```python
from build123d import *

# Parameters (mm, degrees)
ESBO_O6_W                = 100
ESBO_O6_H                = 400
RESSALTO_EXTRUS_O2_DEPTH = 18
CORTE_EXTRUS_O2_DEPTH    = 413.703283244
ESBO_O8_R                = 1.5
CORTE_EXTRUS_O3_DEPTH    = 413.703283244


with BuildPart() as part:
    # Esboço6 → Ressalto-extrusão2 (new body)
    with BuildSketch(Plane.XY):
        with Locations((50, 200)):
            Rectangle(ESBO_O6_W, ESBO_O6_H)
    extrude(amount=RESSALTO_EXTRUS_O2_DEPTH)

    # Esboço7 → Corte-extrusão2 (cut, through all)
    with BuildSketch(Plane.XY.offset(18)):
        Polygon((50, 400), (100, 350), (100, 400), align=None)
        Polygon((100, 50), (50, 0), (100, 0), align=None)
    extrude(amount=-CORTE_EXTRUS_O2_DEPTH, mode=Mode.SUBTRACT)

    # Esboço8 → Corte-extrusão3 (cut, through all)
    with BuildSketch(Plane(origin=(0, 0, 0), x_dir=(-1, 0, 0), z_dir=(0, 0, -1))):
        with Locations((-75, 160)):
            Circle(ESBO_O8_R)
        with Locations((-43, 160)):
            Circle(ESBO_O8_R)
        with Locations((-9, 50)):
            Circle(ESBO_O8_R)
        with Locations((-9, 110)):
            Circle(ESBO_O8_R)
    extrude(amount=-CORTE_EXTRUS_O3_DEPTH, mode=Mode.SUBTRACT)


solid = part.part
```
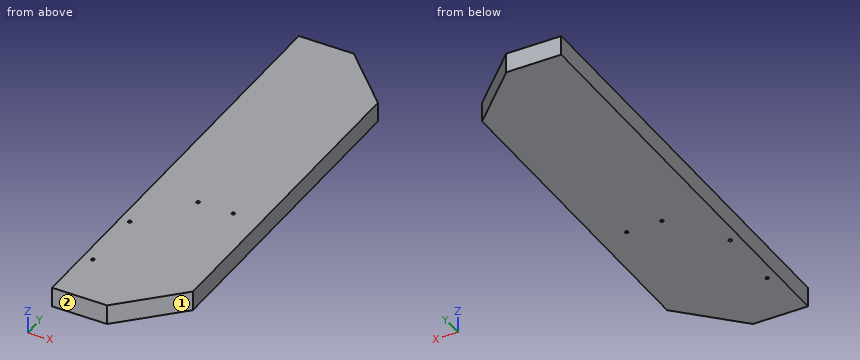
Can you work these out from the model? Positions are in its coordinate system, mm. Face numbers are marked on the shaded views. Coordinates: 2 decimals unless noted, no trailing zeros. Order: outer loops, then holes, each group sorted by start corner. A loop starts at its lowest first (then second) coordinate and runs counter-clockwise, first axis right, second up. Notation, with made-up numbers: (24.5, 76) - (31.5, 76) arc R15 ccw to (31.5, 97) - close; hole circle Ø9 at (-38, -28). An arc over 180 degrees is marked (long way). Answer in a Markdown table with one row per item.
1. Suppose I cut it at B-B (x = 86.5). Please give me the cut outline in (y, z).
Reply:
| item | result |
|---|---|
| outline | (36.5, 0) - (363.5, 0) - (363.5, 18) - (36.5, 18) - close |
2. If we mould it in two halves opening along X, with no side actions, what happens to the marked faces 1 and 2? For each: pulls with the +X half, pulls with the -X half, needs draft (parallel to the pull), parting line crosses it, or undercut.
Reply:
| item | result |
|---|---|
| face 1 | pulls with the +X half |
| face 2 | needs draft |
3. Suppose I cut it at A-A (z = 11.5). Please give me the cut outline in (x, y), and give its area (3 significant figures).
Reply:
| item | result |
|---|---|
| outline | (0, 0) - (50, 0) - (100, 50) - (100, 350) - (50, 400) - (0, 400) - close; hole circle Ø3 at (9, 50); hole circle Ø3 at (9, 110); hole circle Ø3 at (43, 160); hole circle Ø3 at (75, 160) |
| area | 37,500 mm^2 |
4. Suppose I cut it at C-C (x = 68). Please give me the cut outline in (y, z).
Reply:
| item | result |
|---|---|
| outline | (18, 0) - (382, 0) - (382, 18) - (18, 18) - close |
5. For pin 1 (4 mm diameter, centred on x = 63.5, z = 3.5, fed in from +Y); pin 2 (1.8 mm diameter, centred on x = 9, y = 50, fed in from -Z); pin 3 (3 mm diameter, centred on x = 81.5, z = 14, fed in from -Y), each with a flat end and sliding along its axis, tell me the tip position at first contact or that it passes through.
Reply:
| item | result |
|---|---|
| pin 1 | stops at y = 388.5 |
| pin 2 | passes through |
| pin 3 | stops at y = 30 |
6. If I drill on line 1 along X through (y, z) = (160, 7.5); line 2 along Y through (x, z) = (9, 17); line 3 along X through (y, z) = (110, 14), over which ranges is the centre line in solid material (lowest first)?
Reply:
| item | result |
|---|---|
| line 1 | x = 0 to 41.5, 44.5 to 73.5, 76.5 to 100 |
| line 2 | y = 0 to 48.5, 51.5 to 108.5, 111.5 to 400 |
| line 3 | x = 0 to 7.5, 10.5 to 100 |
